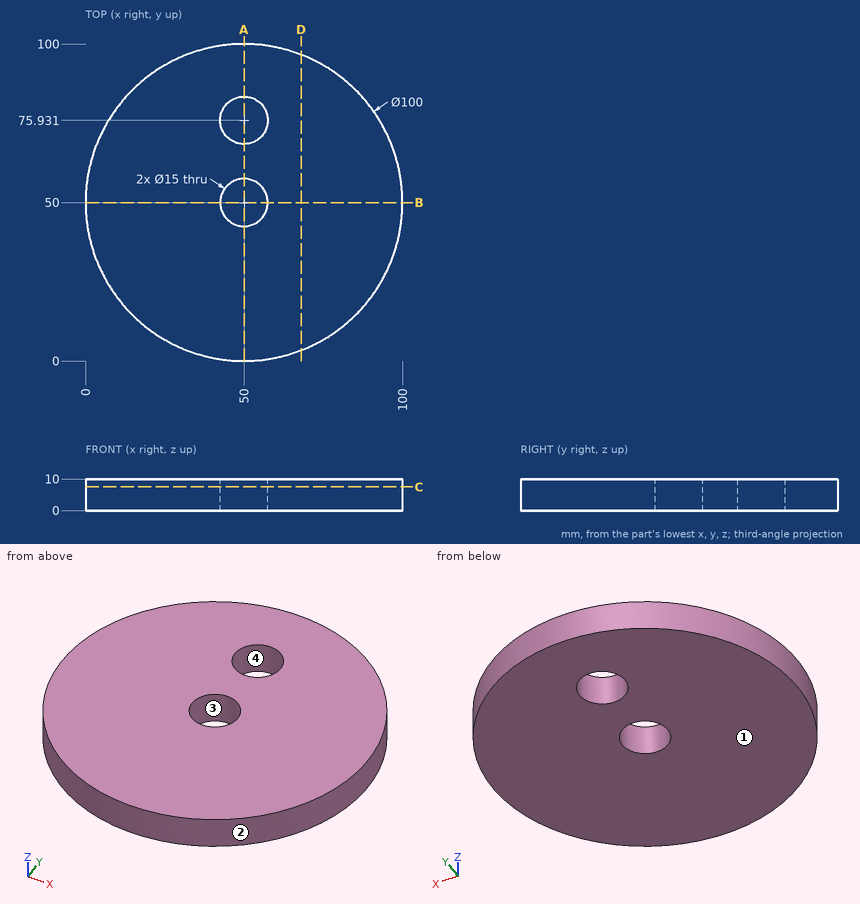
Design review of the part shown in the three views and the two pictorial views. Dimensions are in mm from the part's minimum x, y and z. Round coordinates to 2 decimals unless told otherwise and drop trailing zeros. Loops run counter-clockwise (first coordinate to the right, second up) from the corner with the lowest first, then second, coordinate; pieces in that order, holes last. Notation, with made-up numbers: (32, 63) -> (47, 63) arc R14 ccw to (47, 89) -> close; hole circle Ø5 at (46, -33.5). An arc over 180 degrees is marked (long way). Use one line per item in the form item = value. Start each with the question number.
Q1. We need section D-D on x = 68. Give the boundary of the cut face in (y, z), then the cut area to 3 significant figures.
Q2. We need section B-B on y = 50. Give the boundary of the cut face in (x, z), then the cut area to 3 significant figures.
Q3. For pin 1 Ø2 at (x, z) = (23.5, 1.5) entering from -Y; pin 2 Ø2 at (y, z) = (11, 2) entering from +X (1 decimal); pin 3 Ø1.5 at (x, z) = (81, 6) entering from +Y, all flat-tipped, find the tip position at first contact; note any pin that passes through.
Q4. Draft analysis for pull direction X (two halves, no side actions). For the marked faces 1, 2, 3 and 4, state which applies: +X half, -X half, draft (parallel to the pull), parting line (faces both ways), or undercut.
Q5. We need section A-A on x = 50. Give the boundary of the cut face in (y, z), then the cut area to 3 significant figures.
Q6. We need section C-C on z = 7.5. Give the boundary of the cut face in (x, y), then the cut area to 3 significant figures.
Q7. Wall thickness on line 1 along Y through (x, z) = (50, 7.5); line 2 along Y through (x, z) = (52, 9); line 3 along X through (y, z) = (51.5, 9.75): over which ranges is each line inside the solid? List them lowest first. Write a range as [from, to].
Calculated:
q1.outline = (3.35, 0) -> (96.65, 0) -> (96.65, 10) -> (3.35, 10) -> close
q1.area = 933 mm²
q2.outline = (0, 0) -> (42.5, 0) -> (42.5, 10) -> (0, 10) -> close; (57.5, 0) -> (100, 0) -> (100, 10) -> (57.5, 10) -> close
q2.area = 850 mm²
q3.pin_1 = 6.99
q3.pin_2 = 82.5
q3.pin_3 = 89.81
q4.face_1 = draft
q4.face_2 = parting line
q4.face_3 = undercut
q4.face_4 = undercut
q5.outline = (0, 0) -> (42.5, 0) -> (42.5, 10) -> (0, 10) -> close; (57.5, 0) -> (68.43, 0) -> (68.43, 10) -> (57.5, 10) -> close; (83.43, 0) -> (100, 0) -> (100, 10) -> (83.43, 10) -> close
q5.area = 700 mm²
q6.outline = circle Ø100 at (50, 50); hole circle Ø15 at (50, 50); hole circle Ø15 at (50, 75.93)
q6.area = 7,500 mm²
q7.line_1 = [0, 42.5], [57.5, 68.43], [83.43, 100]
q7.line_2 = [0.04, 42.77], [57.23, 68.7], [83.16, 99.96]
q7.line_3 = [0.02, 42.65], [57.35, 99.98]
